Verification items for this drawing (mm, ordinates from the low corner). A direction names the side the tool comes from. Round coordinates to 2 decimals unless told otherwise and drop trailing zeros. Order: outer loops, then holes, each group sorted by start corner. A loop starts at its lowest first (then second) coordinate and runs counter-clockwise, first axis right, second up. Notation, with made-up numbers: M -36,3.25 L -22,3.25 A13 cw -22,16.25 Z; hole C 29.5,62.5 d2. An arc over 180 degrees is marked long. Return JSON: item names as keys, results as strings. Group by question number.
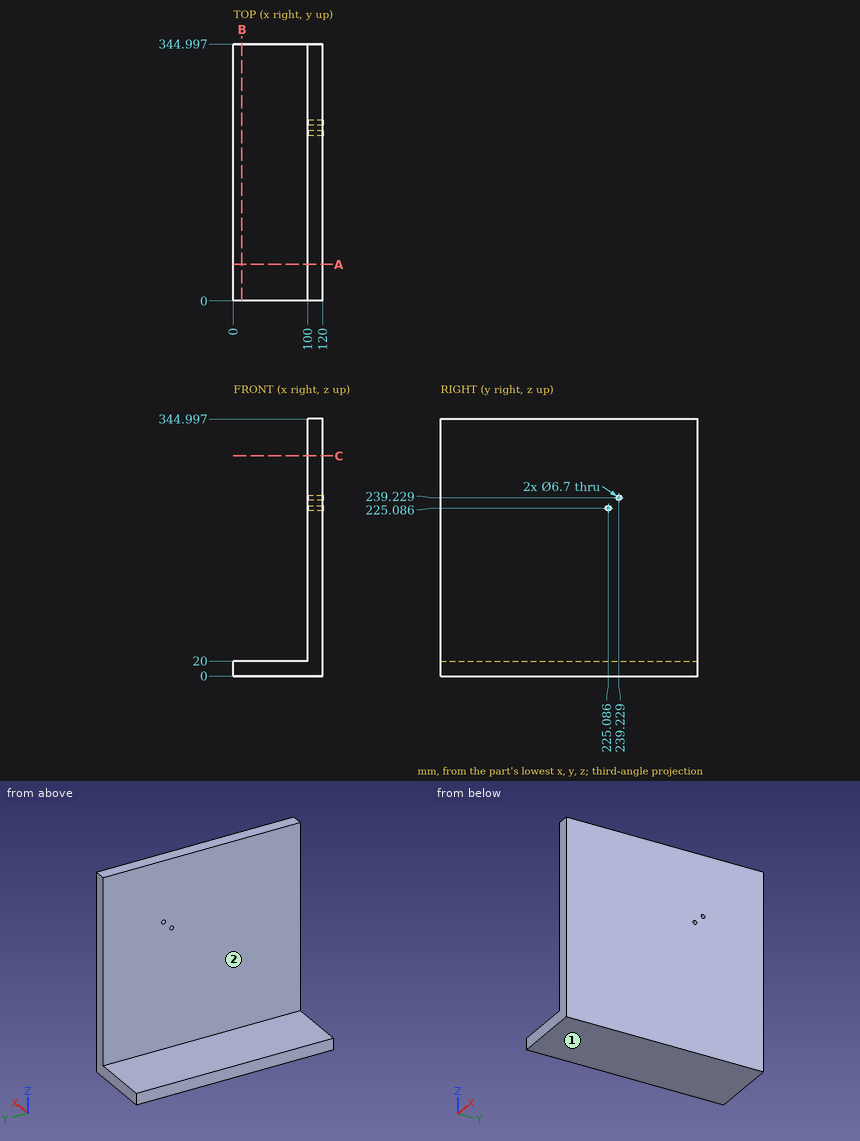
Q1. Section check B-B on x = 11.5. Record the cut outline in (y, z).
Q2. Set-up check for the marked faces 1 and 2: record each of +Z, -Z, +X, -X, +Y, -Y from which the full face is reachable in a straight line by a thin tool's end or side.
Q3. Material ranges on line 1 along X through (y, z) = (123, 102); line 2 along Z through (x, y) = (70, 214); line 3 along Y through (x, z) = (115.5, 240.5), recorded low to high.
Q4. Section check A-A on y = 49. Record the cut outline in (x, z).
Q5. Section check C-C on z = 295.5. Record the cut outline in (x, y).
Q6. Depth check by flat-ended pin: pin 1 Ø2 at (y, z) = (294, 219.5) entering from -X; pin 2 Ø4 at (x, y) = (18, 302.5) entering from +Z. Enter the tip coordinate at first touch or a pass-through.
Geometry check:
{
 "1": {"outline": "M 0,0 L 345,0 L 345,20 L 0,20 Z"},
 "2": {"face 1": "-Z, +X, -X, +Y, -Y", "face 2": "+Z, -X, +Y, -Y"},
 "3": {"line 1": "x = 100 to 120", "line 2": "z = 0 to 20", "line 3": "y = 0 to 236.13, 242.33 to 345"},
 "4": {"outline": "M 0,0 L 120,0 L 120,345 L 100,345 L 100,20 L 0,20 Z"},
 "5": {"outline": "M 100,0 L 120,0 L 120,345 L 100,345 Z"},
 "6": {"pin 1": "stops at x = 100", "pin 2": "stops at z = 20"}
}
